```python
from build123d import *

# Parameters (mm, degrees)
ESBO_O1_W                = 2
ESBO_O1_H                = 11
ESBO_O1_W_2              = 10
ESBO_O1_H_2              = 3
RESSALTO_EXTRUS_O1_DEPTH = 6.5
ESBO_O4_W                = 10
ESBO_O4_H                = 2
RESSALTO_EXTRUS_O2_DEPTH = 62
RESSALTO_EXTRUS_O3_START = -59
ESBO_O4_3_W              = 10
ESBO_O4_3_H              = 2
RESSALTO_EXTRUS_O3_DEPTH = 59
RESSALTO_EXTRUS_O4_DEPTH = 2
RESSALTO_EXTRUS_O5_START = -2
RESSALTO_EXTRUS_O5_DEPTH = 2
ESBO_O8_W                = 16
ESBO_O8_H                = 2
CORTE_EXTRUS_O1_DEPTH    = 10


with BuildPart() as part:
    # Esbo_o1 → Ressalto-extrus_o1 (new body)
    with BuildSketch(Plane.XY):
        Polygon((15, 19), (15, 0), (15, -41), (17, -41), (17, 57), (17, 62), (-17, 62), (-17, 57), (-17, -41), (-15, -41), (-15, 0), (-15, 19), (-15, 27), (-15, 57), (-15, 60), (-5, 60), (0, 60), (5, 60), (15, 60), (15, 57), (15, 27), align=None)
        with Locations((16, -46.5)):
            Rectangle(ESBO_O1_W, ESBO_O1_H)
        Polygon((15, -57), (0, -57), (-15, -57), (-15, -52), (-17, -52), (-17, -59), (17, -59), (17, -52), (15, -52), align=None)
        with Locations((-16, -46.5)):
            Rectangle(ESBO_O1_W, ESBO_O1_H)
        with Locations((10, 58.5)):
            Rectangle(ESBO_O1_W_2, ESBO_O1_H_2)
        with Locations((-10, 58.5)):
            Rectangle(ESBO_O1_W_2, ESBO_O1_H_2)
    extrude(amount=RESSALTO_EXTRUS_O1_DEPTH)

    # Esbo_o4 → Ressalto-extrus_o2 (add)
    with BuildSketch(Plane(origin=(0, 0, 0), x_dir=(1, 0, 0), z_dir=(0, 1, 0))):
        with BuildLine():
            ThreePointArc((-10, 7), (-14.949747468, 4.949747468), (-17, 0))
            Line((-17, 0), (-15, 0))
            ThreePointArc((-15, 0), (-13.535533906, 3.535533906), (-10, 5))
            Line((-10, 5), (-10, 7))
        make_face()
        with Locations((-5, 6)):
            Rectangle(ESBO_O4_W, ESBO_O4_H)
        with BuildLine():
            Line((15, 0), (17, 0))
            ThreePointArc((17, 0), (14.949747468, 4.949747468), (10, 7))
            Line((10, 7), (0, 7))
            Line((0, 7), (0, 5))
            Line((0, 5), (10, 5))
            ThreePointArc((10, 5), (13.535533906, 3.535533906), (15, 0))
        make_face()
    extrude(amount=RESSALTO_EXTRUS_O2_DEPTH)

    # Esbo_o4_3 → Ressalto-extrus_o3 (add)
    with BuildSketch(Plane(origin=(0, 0, 0), x_dir=(1, 0, 0), z_dir=(0, 1, 0)).offset(RESSALTO_EXTRUS_O3_START)):
        with Locations((-5, 6)):
            Rectangle(ESBO_O4_3_W, ESBO_O4_3_H)
        with BuildLine():
            ThreePointArc((-10, 7), (-14.949747468, 4.949747468), (-17, 0))
            Line((-17, 0), (-15, 0))
            ThreePointArc((-15, 0), (-13.535533906, 3.535533906), (-10, 5))
            Line((-10, 5), (-10, 7))
        make_face()
        with BuildLine():
            Line((15, 0), (17, 0))
            ThreePointArc((17, 0), (14.949747468, 4.949747468), (10, 7))
            Line((10, 7), (0, 7))
            Line((0, 7), (0, 5))
            Line((0, 5), (10, 5))
            ThreePointArc((10, 5), (13.535533906, 3.535533906), (15, 0))
        make_face()
    extrude(amount=RESSALTO_EXTRUS_O3_DEPTH)

    # Esbo_o6 → Ressalto-extrus_o4 (add)
    # profile 1 of 2: a face of its own
    with BuildSketch(Plane.XZ.offset(59)):
        with BuildLine():
            Line((-10, -7), (10, -7))
            ThreePointArc((10, -7), (14.949747468, -4.949747468), (17, 0))
            Line((17, 0), (17, 6.5))
            Line((17, 6.5), (-17, 6.5))
            Line((-17, 6.5), (-17, 0))
            ThreePointArc((-17, 0), (-14.949747468, -4.949747468), (-10, -7))
        make_face()
        with BuildLine():
            ThreePointArc((-10, -5), (-13.535533906, -3.535533906), (-15, 0))
            Line((-15, 0), (15, 0))
            ThreePointArc((15, 0), (13.535533906, -3.535533906), (10, -5))
            Line((10, -5), (-10, -5))
        make_face(mode=Mode.SUBTRACT)
    # profile 2 of 2: a face of its own
    with BuildSketch(Plane.XZ.offset(59)):
        with BuildLine():
            Line((-15, 0), (15, 0))
            ThreePointArc((15, 0), (13.535533906, -3.535533906), (10, -5))
            Line((10, -5), (-10, -5))
            ThreePointArc((-10, -5), (-13.535533906, -3.535533906), (-15, 0))
        make_face()
    extrude(amount=-RESSALTO_EXTRUS_O4_DEPTH)

    # Esbo_o7 → Ressalto-extrus_o5 (add)
    with BuildSketch(Plane(origin=(0, 62, 0), x_dir=(1, 0, 0), z_dir=(0, 1, 0)).offset(RESSALTO_EXTRUS_O5_START)):
        with BuildLine():
            Line((17, 0), (17, -6.5))
            Line((17, -6.5), (-17, -6.5))
            Line((-17, -6.5), (-17, 0))
            ThreePointArc((-17, 0), (-14.949747468, 4.949747468), (-10, 7))
            Line((-10, 7), (10, 7))
            ThreePointArc((10, 7), (14.949747468, 4.949747468), (17, 0))
        make_face()
    extrude(amount=RESSALTO_EXTRUS_O5_DEPTH)

    # Esbo_o8 → Corte-extrus_o1 (cut, symmetric)
    with BuildSketch(Plane(origin=(0, 0, -7), x_dir=(-1, 0, 0), z_dir=(0, 0, -1))):
        with Locations((0, 53)):
            Rectangle(ESBO_O8_W, ESBO_O8_H)
        with Locations((0, 49)):
            Rectangle(ESBO_O8_W, ESBO_O8_H)
        with Locations((0, 45)):
            Rectangle(ESBO_O8_W, ESBO_O8_H)
        with Locations((0, 41)):
            Rectangle(ESBO_O8_W, ESBO_O8_H)
        with Locations((0, 37)):
            Rectangle(ESBO_O8_W, ESBO_O8_H)
        with Locations((0, 33)):
            Rectangle(ESBO_O8_W, ESBO_O8_H)
    extrude(amount=CORTE_EXTRUS_O1_DEPTH, both=True, mode=Mode.SUBTRACT)


solid = part.part
```
Verification items for the finished model (mm, model axes). A direction names the side the tool comes from. Coordinates: 2 decimals unless noted, no trailing zeros. Loops run counter-clockwise (first coordinate to the right, second up) from the corner with the lowest first, then second, coordinate; pieces in that order, holes last. Notation, with made-up numbers: (7, -25) -> (34, -25) arc R25 ccw to (34, 11) -> close; hole circle Ø11 at (-15, -14). An arc over 180 degrees is marked (long way). Answer in a Markdown table with one row per item.
1) Section check D-D (x = 11.5). Record the cut outline in (y, z), and give its area (3 significant figures).
The answers:
| item | result |
|---|---|
| outline | (-59, -6.84) -> (62, -6.84) -> (62, 6.5) -> (57, 6.5) -> (57, 0) -> (60, 0) -> (60, -4.77) -> (-57, -4.77) -> (-57, 6.5) -> (-59, 6.5) -> close |
| area | 315 mm2 |
2) Section check C-C (z = 4.5). Record the cut outline in (x, y), and give its area (3 significant figures).
The answers:
| item | result |
|---|---|
| outline | (-17, -59) -> (17, -59) -> (17, 62) -> (-17, 62) -> close; hole (-15, -57) -> (15, -57) -> (15, 57) -> (5, 57) -> (5, 60) -> (-5, 60) -> (-5, 57) -> (-15, 57) -> close |
| area | 664 mm2 |
3) Section check A-A (x = -2). Give the number of separate pieces and of enclosed holes in the cut face, and give its area (3 significant figures).
The answers:
| item | result |
|---|---|
| separate pieces | 7 |
| enclosed holes | 0 |
| area | 264 mm2 |
4) Access from +Z, -Z, +X, -X, +Y, -Y to the whole of each face (thin tool, end or side, straight path). Record for faces 1 (the face through (-5, 58, 3)), 2 (the face through (0, 1, -7)), 3 (the face through (10, 59, 0)), 4 (the face through (8, 53, -6)).
The answers:
| item | result |
|---|---|
| face 1 | +Z |
| face 2 | -Z, +X, -X, +Y, -Y |
| face 3 | none |
| face 4 | +Z, -Z |
5) Scan lines: line 1 along Y through (x, z) = (-14, -1.5); line 2 along X through (y, z) = (1, 1); line 3 along Y through (x, z) = (6, 2.25). Record each from-to range of solid material in increasing order. Write a range as from..to.
The answers:
| item | result |
|---|---|
| line 1 | y = -59..-57, 60..62 |
| line 2 | x = -17..-15, 15..17 |
| line 3 | y = -59..-57, 57..62 |
6) Section check B-B (y = -16). Record the cut outline in (x, z), and give its area (3 significant figures).
The answers:
| item | result |
|---|---|
| outline | (-17, 0) arc R7 ccw to (-10, -7) -> (10, -7) arc R7 ccw to (17, 0) -> (17, 6.5) -> (15, 6.5) -> (15, 0) arc R5 cw to (10, -5) -> (-10, -5) arc R5 cw to (-15, 0) -> (-15, 6.5) -> (-17, 6.5) -> close |
| area | 104 mm2 |
7) Depth check by flat-ended pin: P1, Ø0.6, axis at y = 49.5, z = -5.5, coming from the +X side; P2, Ø1, axis at y = 45, z = -5.5, coming from the +X side; P3, Ø2, axis at y = 36.5, z = -5.5, coming from the -X side; P4, Ø6, axis at x = 13, y = -3.5, coming from the +Z side. Enter the tip coordinate at first touch or a pass-through.
The answers:
| item | result |
|---|---|
| P1 | stops at x = 14.69 |
| P2 | stops at x = 14.9 |
| P3 | stops at x = -15.36 |
| P4 | stops at z = 6.5 |
8) Draft check along Y on faces 5 (the face through (8, 45, -6)), 6 (the face through (8, 49, -6)), 7 (the face through (17, 1, 3)). Enter one of: released by +Y, released by -Y, zero draft, split by the parting line, or undercut.
The answers:
| item | result |
|---|---|
| face 5 | undercut |
| face 6 | undercut |
| face 7 | zero draft |
